```python
from build123d import *

# Parameters (mm, degrees)
F0_W     = 20
F0_H     = 10
F1_DEPTH = 5
F2_R     = 1
F3_DEPTH = 10


with BuildPart() as f1:
    # F0 (on Top) → F1 (new body)
    with BuildSketch(Plane.XY):
        Rectangle(F0_W, F0_H)
    extrude(amount=F1_DEPTH)

    # F2 (on face) → F3 (cut, through all)
    with BuildSketch(Plane.XZ.offset(5)):
        with Locations((-5, 2.5)):
            Circle(F2_R)
        with Locations((0, 2.5)):
            Circle(F2_R)
        with Locations((5, 2.5)):
            Circle(F2_R)
    extrude(amount=-F3_DEPTH, mode=Mode.SUBTRACT)


solid = f1.part
```
Check sheet for the modelled part. Datum: model origin and axes. Units: mm. Give positions to 0.01 mm unless a question says otherwise; leave off trailing zeros. Loops run counter-clockwise (first coordinate to the right, second up) from the corner with the lowest first, then second, coordinate; pieces in that order, holes last. Notation, with made-up numbers: M 39.25,-25.75 L 74.25,-25.75 A31 cw 74.25,9.25 Z; hole C 76,3 d8. An arc over 180 degrees is marked long. Answer as CSV lines item,"result".
Item 1: Draft check along Z on faces 1 (the face through (-6, -0.1, 2.5)), 2 (the face through (-10, 0, 2)), 3 (the face through (0, 0, 0)). Enter one of: pulls with the +Z half, pulls with the -Z half, needs draft (parallel to the pull), parting line crosses it, or undercut.
Reply:
face 1,"undercut"
face 2,"needs draft"
face 3,"pulls with the -Z half"
Item 2: Sectioned sample at D-D, the plane x = -5.25. Enter the section's corners in (y, z), then the cut area to 3 significant figures.
Reply:
outline,"M -5,0 L 5,0 L 5,1.53 L -5,1.53 Z; M -5,3.47 L 5,3.47 L 5,5 L -5,5 Z"
area,"30.6 mm^2"
Item 3: Scan lines: L1, parallel to X at y = 2.5, z = 2.4; L2, parallel to Z at x = 5, y = 3.25; L3, parallel to X at y = -3.5, z = 2. Record each from-to range of solid material in increasing order.
Reply:
L1,"-10 to -5.99, -4.01 to -0.99, 0.99 to 4.01, 5.99 to 10"
L2,"0 to 1.5, 3.5 to 5"
L3,"-10 to -5.87, -4.13 to -0.87, 0.87 to 4.13, 5.87 to 10"
Item 4: Sectioned sample at A-A, the plane x = 5. Enter the section's corners in (y, z).
Reply:
outline,"M -5,0 L 5,0 L 5,1.5 L -5,1.5 Z; M -5,3.5 L 5,3.5 L 5,5 L -5,5 Z"
Item 5: Sectioned sample at C-C, the plane z = 1.75. Enter the section's corners in (x, y).
Reply:
outline,"M -10,-5 L -5.66,-5 L -5.66,5 L -10,5 Z; M -4.34,-5 L -0.66,-5 L -0.66,5 L -4.34,5 Z; M 0.66,-5 L 4.34,-5 L 4.34,5 L 0.66,5 Z; M 5.66,-5 L 10,-5 L 10,5 L 5.66,5 Z"
Item 6: Sectioned sample at B-B, the plane y = 1. Enter the section's corners in (x, z).
Reply:
outline,"M -10,0 L 10,0 L 10,5 L -10,5 Z; hole C -5,2.5 d2; hole C 0,2.5 d2; hole C 5,2.5 d2"
